```python
from build123d import *

# Parameters (mm, degrees)
CROQUIS1_W              = 190
CROQUIS1_H              = 130
SALIENTE_EXTRUIR1_DEPTH = 1
CROQUIS9_R              = 1.25
CROQUIS9_R_2            = 1.5
CORTAR_EXTRUIR2_DEPTH   = 10
CORTAR_EXTRUIR3_REACH   = 3
CORTAR_EXTRUIR4_REACH   = 3


with BuildPart() as part:
    # Croquis1 → Saliente-Extruir1 (new body)
    with BuildSketch(Plane.XY):
        Rectangle(CROQUIS1_W, CROQUIS1_H)
    extrude(amount=SALIENTE_EXTRUIR1_DEPTH)

    # Croquis9 → Cortar-Extruir2 (cut)
    with BuildSketch(Plane(origin=(0, 0, 0), x_dir=(-1, 0, 0), z_dir=(0, 0, -1))):
        with Locations((-44.45, 51)):
            Circle(CROQUIS9_R)
        with Locations((35.357472454, 3.746718702)):
            Circle(CROQUIS9_R_2)
        with Locations((36.270123649, 51.127714796)):
            Circle(CROQUIS9_R_2)
        with Locations((-14.524931807, 18.747519864)):
            Circle(CROQUIS9_R_2)
        with Locations((-14.700351259, 45.987329572)):
            Circle(CROQUIS9_R_2)
        with Locations((-38.24, 3.75)):
            Circle(CROQUIS9_R_2)
    extrude(amount=-CORTAR_EXTRUIR2_DEPTH, mode=Mode.SUBTRACT)

    # Croquis12 → Cortar-Extruir3 (cut, up to next)
    with BuildSketch(Plane(origin=(0, 0, 0), x_dir=(-1, 0, 0), z_dir=(0, 0, -1)), mode=Mode.PRIVATE) as cortar_extruir3_sk1:
        Polygon((-95, 65), (-95, 43.5), (-41.651647359, 65), align=None)
    cortar_extruir3_tool1 = extrude(cortar_extruir3_sk1.sketch, amount=-CORTAR_EXTRUIR3_REACH, mode=Mode.PRIVATE) & part.part
    add(cortar_extruir3_tool1.solids().sort_by_distance((77.217216, 57.833333, 0))[0], mode=Mode.SUBTRACT)
    # Croquis12 → Cortar-Extruir3 (cut, up to next)
    with BuildSketch(Plane(origin=(0, 0, 0), x_dir=(-1, 0, 0), z_dir=(0, 0, -1)), mode=Mode.PRIVATE) as cortar_extruir3_sk2:
        Polygon((41.651647359, 65), (95, 65), (95, 43.5), align=None)
    cortar_extruir3_tool2 = extrude(cortar_extruir3_sk2.sketch, amount=-CORTAR_EXTRUIR3_REACH, mode=Mode.PRIVATE) & part.part
    add(cortar_extruir3_tool2.solids().sort_by_distance((-77.217216, 57.833333, 0))[0], mode=Mode.SUBTRACT)

    # Croquis13 → Cortar-Extruir4 (cut, up to next)
    with BuildSketch(Plane(origin=(0, 0, 0), x_dir=(-1, 0, 0), z_dir=(0, 0, -1)), mode=Mode.PRIVATE) as cortar_extruir4_sk1:
        Polygon((-68.123188454, 42.482226287), (-72.77455345, 52.45711071), (-95, 43.5), (-95.030741331, 42.482226287), align=None)
    cortar_extruir4_tool1 = extrude(cortar_extruir4_sk1.sketch, amount=-CORTAR_EXTRUIR4_REACH, mode=Mode.PRIVATE) & part.part
    add(cortar_extruir4_tool1.solids().sort_by_distance((79.331365, 45.833261, 0))[0], mode=Mode.SUBTRACT)
    # Croquis13 → Cortar-Extruir4 (cut, up to next)
    with BuildSketch(Plane(origin=(0, 0, 0), x_dir=(-1, 0, 0), z_dir=(0, 0, -1)), mode=Mode.PRIVATE) as cortar_extruir4_sk2:
        Polygon((-44.909770717, 63.686938795), (-40.531538935, 54.297790439), (-36, 56.410881748), (-15, 56.410881748), (-15, 65), (-41.651647359, 65), align=None)
    cortar_extruir4_tool2 = extrude(cortar_extruir4_sk2.sketch, amount=-CORTAR_EXTRUIR4_REACH, mode=Mode.PRIVATE) & part.part
    add(cortar_extruir4_tool2.solids().sort_by_distance((29.368606, 60.647773, 0))[0], mode=Mode.SUBTRACT)
    # Croquis13 → Cortar-Extruir4 (cut, up to next)
    with BuildSketch(Plane(origin=(0, 0, 0), x_dir=(-1, 0, 0), z_dir=(0, 0, -1)), mode=Mode.PRIVATE) as cortar_extruir4_sk3:
        Polygon((44.909770717, 63.686938795), (41.651647359, 65), (15.011500088, 65), (15, 56.410881748), (36, 56.410881748), (40.531538935, 54.297790439), align=None)
    cortar_extruir4_tool3 = extrude(cortar_extruir4_sk3.sketch, amount=-CORTAR_EXTRUIR4_REACH, mode=Mode.PRIVATE) & part.part
    add(cortar_extruir4_tool3.solids().sort_by_distance((-29.371465, 60.647477, 0))[0], mode=Mode.SUBTRACT)
    # Croquis13 → Cortar-Extruir4 (cut, up to next)
    with BuildSketch(Plane(origin=(0, 0, 0), x_dir=(-1, 0, 0), z_dir=(0, 0, -1)), mode=Mode.PRIVATE) as cortar_extruir4_sk4:
        Polygon((72.77455345, 52.45711071), (68.123188454, 42.482226287), (95, 42.482226287), (95, 43.5), align=None)
    cortar_extruir4_tool4 = extrude(cortar_extruir4_sk4.sketch, amount=-CORTAR_EXTRUIR4_REACH, mode=Mode.PRIVATE) & part.part
    add(cortar_extruir4_tool4.solids().sort_by_distance((-79.329677, 45.833585, 0))[0], mode=Mode.SUBTRACT)


solid = part.part
```
Build history of the part. All positions in model axes, mm. A direction names the side the tool comes from. Give positions to 0.01 mm unless a question says otherwise; leave off trailing zeros. Loops run counter-clockwise (first coordinate to the right, second up) from the corner with the lowest first, then second, coordinate; pieces in that order, holes last. Notation, with made-up numbers: (88, 7) - (108, 7) arc R16 cw to (108, 24) - close; hole circle Ø11 at (25.5, 56.5). An arc over 180 degrees is marked (long way). Use a Markdown table: item, result.
(1) Band-saw the part on B-B (x = -77). Give the cut face in (y, z), and give its area (3 significant figures).
Taken from the geometry:
| item | result |
|---|---|
| outline | (-65, 0) - (42.48, 0) - (42.48, 1) - (-65, 1) - close |
| area | 107 mm2 |
(2) Drop flat-ended pins along their axis: pin 1 Ø2.5 at (x, y) = (14.52, 18.75) entering from +Z; pin 2 Ø0.5 at (x, z) = (75.5, 0.5) entering from +Y; pin 3 Ø0.5 at (x, z) = (23.5, 0.5) entering from +Y. Give the stop position or say it passes through.
Taken from the geometry:
| item | result |
|---|---|
| pin 1 | through |
| pin 2 | y = 42.48 |
| pin 3 | y = 56.41 |
(3) Which spindle directions (+Z, -Z, +X, -X, +Y, -Y) get a long thin tool onto all of the face, cutting with end or side? Do faces 1 (the face through (70.416, 47.4, 0.493)), 2 (the face through (-70.48, 47.54, 0.49)), 3 (the face through (-42.69, 58.93, 0.49)). Say none if no direction does.
Taken from the geometry:
| item | result |
|---|---|
| face 1 | +Z, -Z, +X |
| face 2 | +Z, -Z, -X |
| face 3 | +Z, -Z, +Y |
(4) Pull direction X, two halves, no side cores. Call faces 4 (the face through (59.037, 57.993, 0.493)), 5 (the face through (42.75, 59.06, 0.49)), 6 (the face through (-1, 1, 1)): +X half, -X half, draft (parallel to the pull), parting line (faces both ways), or undercut.
Taken from the geometry:
| item | result |
|---|---|
| face 4 | +X half |
| face 5 | undercut |
| face 6 | draft |
(5) Wall check: line 1 along X through (y, z) = (56.5, 0.75); line 2 along Y through (x, z) = (-79, 0.5); line 3 along Y through (x, z) = (-24, 0.3). Give the ranges that are in metal, low to high.
Taken from the geometry:
| item | result |
|---|---|
| line 1 | -62.74 to -41.56, -15 to 15, 41.56 to 62.74 |
| line 2 | -65 to 42.48 |
| line 3 | -65 to 56.41 |
(6) Band-saw the part on A-A (z = 0.8). Give the cut face in (x, y).
Taken from the geometry:
| item | result |
|---|---|
| outline | (-95, -65) - (95, -65) - (95, 42.48) - (68.12, 42.48) - (72.77, 52.46) - (44.91, 63.69) - (40.53, 54.3) - (36, 56.41) - (15, 56.41) - (15, 65) - (-15.01, 65) - (-15, 56.41) - (-36, 56.41) - (-40.53, 54.3) - (-44.91, 63.69) - (-72.77, 52.46) - (-68.12, 42.48) - (-95, 42.48) - close; hole circle Ø3 at (-36.27, 51.13); hole circle Ø3 at (-35.36, 3.75); hole circle Ø3 at (14.52, 18.75); hole circle Ø3 at (14.7, 45.99); hole circle Ø3 at (38.24, 3.75); hole circle Ø2.5 at (44.45, 51) |
